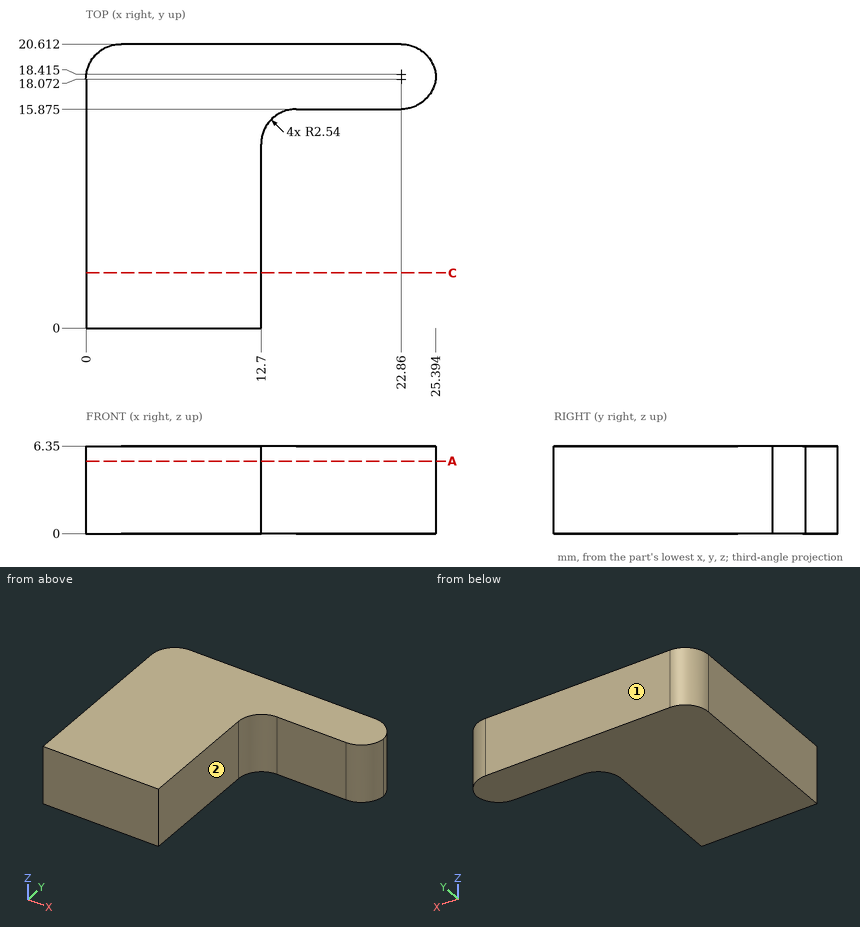
Source: three-view drawing plus pictorial views. Frame: mm from the lowest corner of the part. A direction names the side the tool comes from. Round coordinates to 2 decimals unless told otherwise and drop trailing zeros. Order: outer loops, then holes, each group sorted by start corner. A loop starts at its lowest first (then second) coordinate and runs counter-clockwise, first axis right, second up. Notation, with made-up numbers: (52.25, -29.5) - (80.25, -29.5) arc R19 ccw to (80.25, 1.5) - close; hole circle Ø11 at (55.25, 25.25). An arc over 180 degrees is marked (long way). Use a Markdown table: item, result.
1. Material intervals for probe 1 along X at (y, z) = (6.5, 2); probe 2 along Y at (x, z) = (16.5, 4.75) (1 decimal); probe 3 along Y at (x, z) = (2.25, 2.25) (1 decimal), sorted ascending.
Evaluation:
| item | result |
|---|---|
| probe 1 | 0 to 12.7 |
| probe 2 | 15.9 to 20.6 |
| probe 3 | 0 to 20.6 |
2. First-contact query: pin 1 (1 mm diameter, centred on y = 7.5, z = 2.5, fed in from +X); pin 2 (3 mm diameter, centred on x = 18, z = 4.5, fed in from -Y) (3 decimals). Flat tips, straight axial feed; report the tip coordinate or a pass-through.
Evaluation:
| item | result |
|---|---|
| pin 1 | x = 12.7 |
| pin 2 | y = 15.875 |
3. Section C-C on y = 4. Return the cut outline in (x, z).
Evaluation:
| item | result |
|---|---|
| outline | (0, 0) - (12.7, 0) - (12.7, 6.35) - (0, 6.35) - close |
4. Access query for the marked faces 1 and 2. Directions: +Z, -Z, +X, -X, +Y, -Y. A direction counts if a zero-diameter tool reaches every point of the face in a straight line with its end or side. Return the directions, or none.
Evaluation:
| item | result |
|---|---|
| face 1 | +Z, -Z, +X, -X, +Y |
| face 2 | +Z, -Z, +X, -Y |
5. Section A-A on z = 5.25. Return the cut outline in (x, y) (1 decimal), then the cut area to 3 significant figures.
Evaluation:
| item | result |
|---|---|
| outline | (0, 0) - (12.7, 0) - (12.7, 13.3) arc R2.5 cw to (15.2, 15.9) - (22.9, 15.9) arc R2.5 ccw to (25.4, 18.2) arc R2.5 ccw to (22.9, 20.6) - (2.5, 20.6) arc R2.5 ccw to (0, 18.1) - close |
| area | 319 mm^2 |
